Read the model definition and answer for the solid it produces. Units are mm, in the model's axes. A direction names the side the tool comes from. Coordinates: 2 decimals unless noted, no trailing zeros. Write each loop counter-clockwise with the first axis right and the second up, starting at its lowest first coordinate (ties: lowest second). Pieces come first, ordered by that corner, then holes.
(1) Given pin 1 (1.5 mm diameter, centred on x = 55.5, z = 5, fed in from +Y), flat-ended and moving along its own axis, determine where the tip first touches the part or whether it passes through.
(2) The part is cut by section C-C, the plane y = 20.5. Determine the outline of the cut face in (x, z), and give its area (3 significant figures).
(3) The part is cut by section A-A, the plane x = 140.5. Determine the outline of the cut face in (y, z).
(4) Which of the six approach directions +Z, -Z, +X, -X, +Y, -Y give full straight-line access (tool end or side, diameter ignored) to faces 1 (the flat face through (3, 3.2, 1)), 2 (the flat face through (-205.5, 7, 13))?
(5) The part is cut by section B-B, the plane z = 5.75. Determine the outline of the cut face in (x, y), and give its area (3 significant figures).
(6) Straight lines are drawn through the part: line 1 along Y through (x, z) = (30, 1.5); line 2 along Z through (x, y) = (-176, 22); line 3 along X through (y, z) = (2.5, 10.75). For each, find the intervals that lie inside material, in ascending order.
```python
from build123d import *

# Parameters (mm, degrees)
F1_DEPTH = 212.5
F3_DEPTH = 25.4


# Not quite as in the source:
# - a pattern or mirror of a feature is missing from the dataset's text; its kind, count and spacing are read off the source's solid


with BuildPart() as f1:
    # F0 (on Right) → F1 (new body, symmetric)
    with BuildSketch(Plane.YZ):
        Polygon((0, 15.2755248485), (0, -10.1244751515), (3.2, -10.1244751515), (3.2, 12.0755248485), (25.4, 12.0755248485), (25.4, 15.2755248485), align=None)
    extrude(amount=F1_DEPTH, both=True)

    # F2 (on face) → F3 (cut)
    with BuildSketch(Plane.XY.offset(15.2755248485)):
        Polygon((-212.5, 25.4), (-212.5, 0), (-187.1, 25.4), align=None)
    f3 = extrude(amount=-F3_DEPTH, mode=Mode.SUBTRACT)

    # F3_copies: F3 across plane
    add(f3.mirror(Plane(origin=(0, 0, 0), x_dir=(0, 0, 1), z_dir=(1, 0, 0))), mode=Mode.SUBTRACT)


solid = f1.part
```
Computed:
1. pin 1: stops at y = 3.2
2. outline: (-192, 12.08) - (192, 12.08) - (192, 15.28) - (-192, 15.28) - close
2. area: 1,230 mm2
3. outline: (0, -10.12) - (3.2, -10.12) - (3.2, 12.08) - (25.4, 12.08) - (25.4, 15.28) - (0, 15.28) - close
4. face 1: -Z, +X, -X, +Y
4. face 2: +Z, -Z, -X, +Y
5. outline: (-212.5, 0) - (212.5, 0) - (209.3, 3.2) - (-209.3, 3.2) - close
5. area: 1,350 mm2
6. line 1: y = 0 to 3.2
6. line 2: z = 12.08 to 15.28
6. line 3: x = -210 to 210
